Can you work these out from the model? Positions are in its coordinate system, mm. A direction names the side the tool comes from. Round coordinates to 2 decimals unless told otherwise and drop trailing zeros.
from build123d import *

# Parameters (mm, degrees)
SKETCH3_R          = 21.166666667
GEARBODY_DEPTH     = 19.05
TOOTHCUT_DEPTH     = 20.05
CIRPATTERN1_COUNT  = 18
BOREDIA_R          = 7.9375
BORE_DEPTH         = 12700
CUT_EXTRUDE1_DEPTH = 20.05


with BuildPart() as part:
    # Sketch3 → gearBody (new body)
    with BuildSketch(Plane.XY):
        Circle(SKETCH3_R)
    extrude(amount=GEARBODY_DEPTH)

    # Sketch2 → toothCut (cut, through all)
    with BuildSketch(Plane.XY):
        with BuildLine():
            ThreePointArc((16.335269031, -2.015998593), (16.377127438, -1.641633799), (16.410407448, -1.266409111))
            ThreePointArc((16.410407448, -1.266409111), (16.667413848, -0.726792607), (17.219915542, -0.498801072))
            ThreePointArc((17.219915542, -0.498801072), (20.650307967, 0.417339666), (23.283949955, 2.798691365))
            ThreePointArc((23.283949955, 2.798691365), (23.334606399, -2.339047473), (22.265196368, -7.364511495))
            ThreePointArc((22.265196368, -7.364511495), (20.156614608, -4.507802025), (16.976312891, -2.929009122))
            ThreePointArc((16.976312891, -2.929009122), (16.480056536, -2.595890687), (16.335269031, -2.015998593))
        make_face()
    toothcut = extrude(amount=TOOTHCUT_DEPTH, mode=Mode.SUBTRACT)

    # CirPattern1: toothCut ×18 about axis
    cirpattern1_axis = Axis((0, 0, 0), (0, 0, 1))
    for i in range(1, CIRPATTERN1_COUNT):
        add(toothcut.rotate(cirpattern1_axis, i * 360 / CIRPATTERN1_COUNT), mode=Mode.SUBTRACT)

    # boreDia → bore (cut, symmetric)
    with BuildSketch(Plane.XY):
        Circle(BOREDIA_R)
    extrude(amount=BORE_DEPTH, both=True, mode=Mode.SUBTRACT)

    # Sketch4 → Cut-Extrude1 (cut, through all)
    with BuildSketch(Plane(origin=(0, 0, 0), x_dir=(-1, 0, 0), z_dir=(0, 0, -1))):
        with BuildLine():
            Line((0, 10.31875), (2.38125, 10.31875))
            Line((2.38125, 10.31875), (2.38125, 7.571892411))
            ThreePointArc((2.38125, 7.571892411), (0, 7.9375), (-2.38125, 7.571892411))
            Line((-2.38125, 7.571892411), (-2.38125, 10.31875))
            Line((-2.38125, 10.31875), (0, 10.31875))
        make_face()
    extrude(amount=-CUT_EXTRUDE1_DEPTH, mode=Mode.SUBTRACT)


solid = part.part
(1) On a 3-axis mill with a long thin cutter (end or side, diameter ignored), from which of +Z, -Z, +X, -X, +Y, -Y can I reach the whole of each face in a straight line? I mean faces 1 (the face through (0, -9, 0)), 2 (the face through (-3.51, -18.92, 9.39)), 3 (the face through (12.15, -15, 9.39)), 4 (the face through (9.47, -16.75, 9.39)), 5 (the face through (-3.17, 18.98, 9.39)). Say none if no direction works.
(2) I'm going to push flat-ended pins straight in: pin 1 Ø8 at (y, z) = (11, 17) entering from +X; pin 2 Ø1.4 at (y, z) = (8.5, 7) entering from -X; pin 3 Ø2 at (y, z) = (9.5, 9.5) entering from +X (3 decimals); pin 4 Ø1.5 at (x, y) = (6.5, 17) entering from -Z. Where does each tip first touch, or does it pass through?
(3) If we mould it in two halves opening along Y, with no side actions, what happens to faces 6 (the face through (2.381, 9, 9)), 7 (the face through (-7.696, 14.795, 9.392)), 8 (the face through (7.696, -14.795, 9.392))? For each: pulls with the +Y half, pulls with the -Y half, needs draft (parallel to the pull), parting line crosses it, or undercut.
(4) Please list where these lines run through material, in increasing order: probe 1 along Y at (x, z) = (-19, 4.75); probe 2 along X at (y, z) = (-12, 17); probe 3 along X at (y, z) = (-18, 2.75).
Ans:
1. face 1: -Z, +X, -X, +Y, -Y
1. face 2: +Z, -Z
1. face 3: +Z, -Z, +X
1. face 4: +Z, -Z, -Y
1. face 5: +Z, -Z, +Y
2. pin 1: stops at x = 19.63
2. pin 2: stops at x = -15.81
2. pin 3: stops at x = 19.385
2. pin 4: stops at z = 0
3. face 6: undercut
3. face 7: pulls with the +Y half
3. face 8: pulls with the -Y half
4. probe 1: y = -9.33 to -7.17, -3.03 to 0.24, 3.71 to 6.73
4. probe 2: x = -14.69 to 11.27, 13.65 to 17.44
4. probe 3: x = -9.96 to -6.9, -3.57 to -0.01, 2.76 to 6.28
